Input: dimensioned drawing with shaded views. Units: mm. Origin: part minimum x, y, z. A direction names the side the tool comes from. Round coordinates to 2 decimals unless told otherwise and drop trailing zeros. Order: outer loops, then holes, each group sorted by start corner. A loop starts at its lowest first (then second) coordinate and runs counter-clockwise, first axis right, second up. Notation, with made-up numbers: (31.25, -4.5) - (77.25, -4.5) arc R20 cw to (77.25, 30.5) - close; hole circle Ø11 at (65, -29.75). An arc over 180 degrees is marked (long way). Return JSON: item names as keys, results as strings. Group by question number.
1) Section A-A, the plane z = 20.5. Return loops of the section in (x, y) (1 decimal).
2) Access query for the marked faces 1 and 2. Directions: +Z, -Z, +X, -X, +Y, -Y. A direction counts if a zero-diameter tool reaches every point of the face in a straight line with its end or side. Return the directions, or none.
3) Ray query, line 1 (Y direction, x = 6.5, z = 27.5); line 2 (Z direction, x = 8.5, y = 10.5); line 3 (Y direction, x = 6.5, z = 10) (1 decimal). Return the intervals inside material, ascending. Write a range as from..to.
4) Contact query for flat-ended pins moving along their axis: P1, Ø4, axis at y = 3, z = 43.5, coming from the -X side; P2, Ø1.5, axis at y = 10, z = 67.5, coming from the +X side (1 decimal); P3, Ø5, axis at x = 11.5, z = 37, coming from the -Y side. Output: stop coordinate, or through.
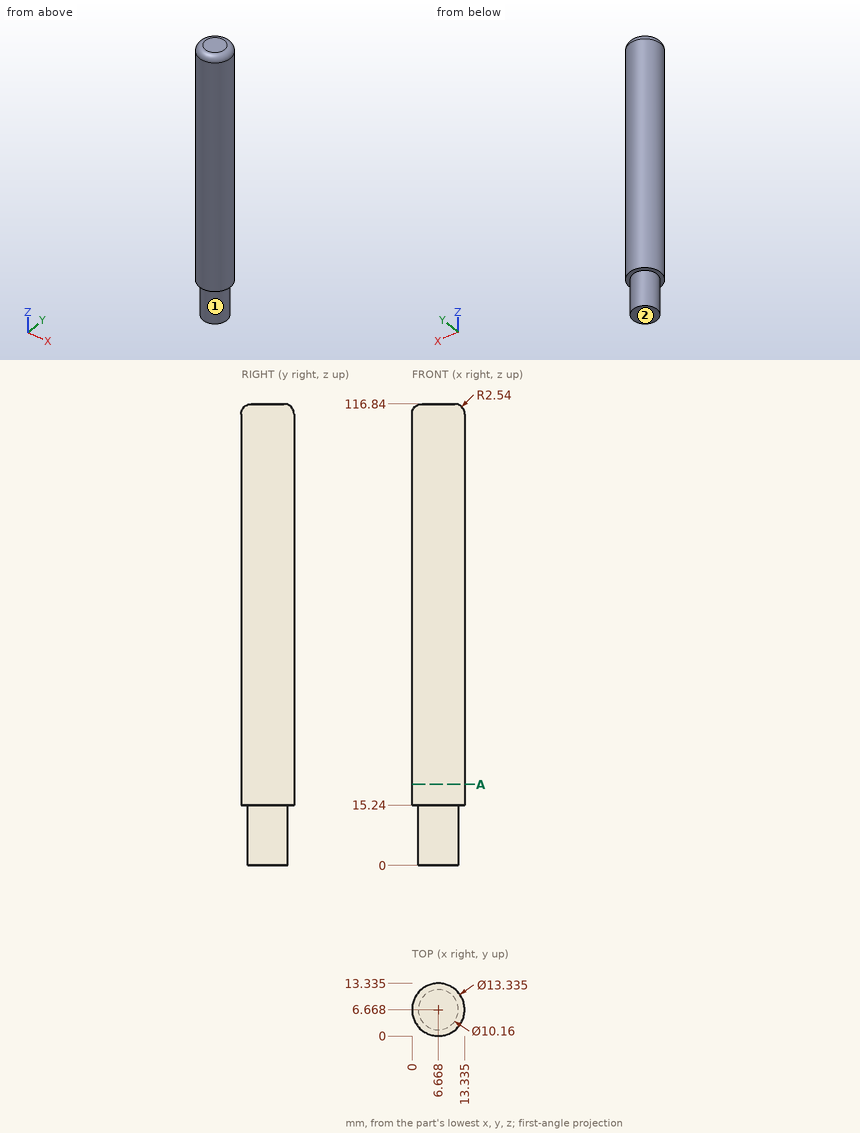
Geometry check:
{
 "1": {"outline": "circle Ø13.3 at (6.7, 6.7)"},
 "2": {"face 1": "-Z", "face 2": "-Z, +X, -X, +Y, -Y"},
 "3": {"line 1": "0..13.33", "line 2": "0..116.84", "line 3": "1.6..11.7"},
 "4": {"P1": "x = 0.21", "P2": "x = 12.8", "P3": "y = 0.42"}
}
